Source: CAD feature listing. Evaluate the final solid. Frame: model axes, mm. Round coordinates to 2 decimals unless told otherwise and drop trailing zeros. Loops run counter-clockwise (first coordinate to the right, second up) from the corner with the lowest first, then second, coordinate; pieces in that order, holes last. Notation, with made-up numbers: (-0.75, 7) - (37.25, 7) arc R29 cw to (37.25, 46) - close; hole circle Ø7 at (-24, -15.5). An arc over 180 degrees is marked (long way). One line per question, with ' | ' between items.
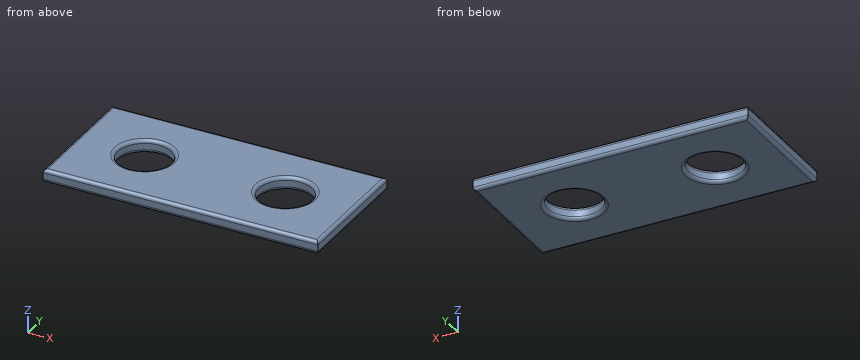
from build123d import *

# Parameters (mm, degrees)
F0_W     = 170
F0_H     = 80
F0_R     = 16.5
F1_DEPTH = 4
F2_R     = 2


with BuildPart() as f1:
    # F0 (on Top) → F1 (new body, symmetric)
    with BuildSketch(Plane.XY):
        Rectangle(F0_W, F0_H)
        with Locations((-43.5, 0)):
            Circle(F0_R, mode=Mode.SUBTRACT)
        with Locations((43.5, 0)):
            Circle(F0_R, mode=Mode.SUBTRACT)
    extrude(amount=F1_DEPTH, both=True)

    # F2
    f2_edges = [f1.edges().sort_by_distance(p)[0] for p in [
        (85, 0, -4),
        (0, 40, -4),
        (-85, 0, -4),
        (0, -40, -4),
        (-60, 0, -4),
        (27, 0, -4),
        (85, 0, 4),
        (0, 40, 4),
        (-85, 0, 4),
        (0, -40, 4),
        (-60, 0, 4),
        (27, 0, 4),
    ]]
    fillet(f2_edges, radius=F2_R)


solid = f1.part
1. Section query B-B, the plane x = -43.5. Return loops of the section in (y, z).
Worked out:
outline: (-40, -2) arc R2 ccw to (-38, -4) - (-18.5, -4) arc R2 ccw to (-16.5, -2) - (-16.5, 2) arc R2 ccw to (-18.5, 4) - (-38, 4) arc R2 ccw to (-40, 2) - close; (16.5, -2) arc R2 ccw to (18.5, -4) - (38, -4) arc R2 ccw to (40, -2) - (40, 2) arc R2 ccw to (38, 4) - (18.5, 4) arc R2 ccw to (16.5, 2) - close
2. Material intervals for probe 1 along Y at (x, z) = (-43.5, -0.5); probe 2 along X at (y, z) = (1.5, -3.5); probe 3 along X at (y, z) = (-12, 1), sorted ascending.
Worked out:
probe 1: y = -40 to -16.5, 16.5 to 40 | probe 2: x = -84.32 to -60.61, -26.39 to 26.39, 60.61 to 84.32 | probe 3: x = -85 to -54.82, -32.18 to 32.18, 54.82 to 85
3. Section query A-A, the plane y = 0. Return loops of the section in (x, z).
Worked out:
outline: (-85, -2) arc R2 ccw to (-83, -4) - (-62, -4) arc R2 ccw to (-60, -2) - (-60, 2) arc R2 ccw to (-62, 4) - (-83, 4) arc R2 ccw to (-85, 2) - close; (-27, -2) arc R2 ccw to (-25, -4) - (25, -4) arc R2 ccw to (27, -2) - (27, 2) arc R2 ccw to (25, 4) - (-25, 4) arc R2 ccw to (-27, 2) - close; (60, -2) arc R2 ccw to (62, -4) - (83, -4) arc R2 ccw to (85, -2) - (85, 2) arc R2 ccw to (83, 4) - (62, 4) arc R2 ccw to (60, 2) - close
